The drawing under review shows one solid part. Ordinate dimensions are in mm from its lowest x, y, z. A direction names the side the tool comes from. Coordinates: 2 decimals unless noted, no trailing zeros. Loops run counter-clockwise (first coordinate to the right, second up) from the corner with the lowest first, then second, coordinate; pieces in that order, holes last. Notation, with made-up numbers: M -35.5,27 L -26.5,27 A23 ccw -26.5,61 Z; hole C 53.5,67 d5. An arc over 180 degrees is marked long. Answer as a JSON object with one key per item and string values. Group by question number.
1. Consider section A-A (z = 23). State the section outline as (x, y) points, then the cut area to 3 significant figures.
2. Insertion check: pin 1 (2 mm diameter, centred on x = 20, z = 36.5, fed in from +Y); pin 2 (0.9 mm diameter, centred on x = 35, y = 1, fed in from +Z); pin 3 (1.6 mm diameter, centred on y = 12, z = 30.5, fed in from -X). Each pin has a flat end and moves straight along its axis. Give the tip position at first contact, or say it passes through.
3. Machinability: for the marked faces 1 and 2, which of the approach directions +Z, -Z, +X, -X, +Y, -Y give a long, thin tool a straight path to every point of the face, cutting with its end or side? Answer none if there is none.
4. Draft analysis for pull direction Z (two halves, no side actions). For the marked faces 3, 4 and 5, state which applies: +Z half, -Z half, draft (parallel to the pull), parting line (faces both ways), or undercut.
5. To check wall thickness, follow probe 1 along Z at (x, y) = (14, 8.75); probe 2 along Z at (x, y) = (13.5, 11.5); probe 3 along X at (y, z) = (5, 30). State the ranges of each line that lie inside material, in increasing order.
6. Consider section B-B (x = 11). State the section outline as (y, z) points.
7. Consider section C-C (y = 1.25). State the section outline as (x, z) points, then the cut area to 3 significant figures.
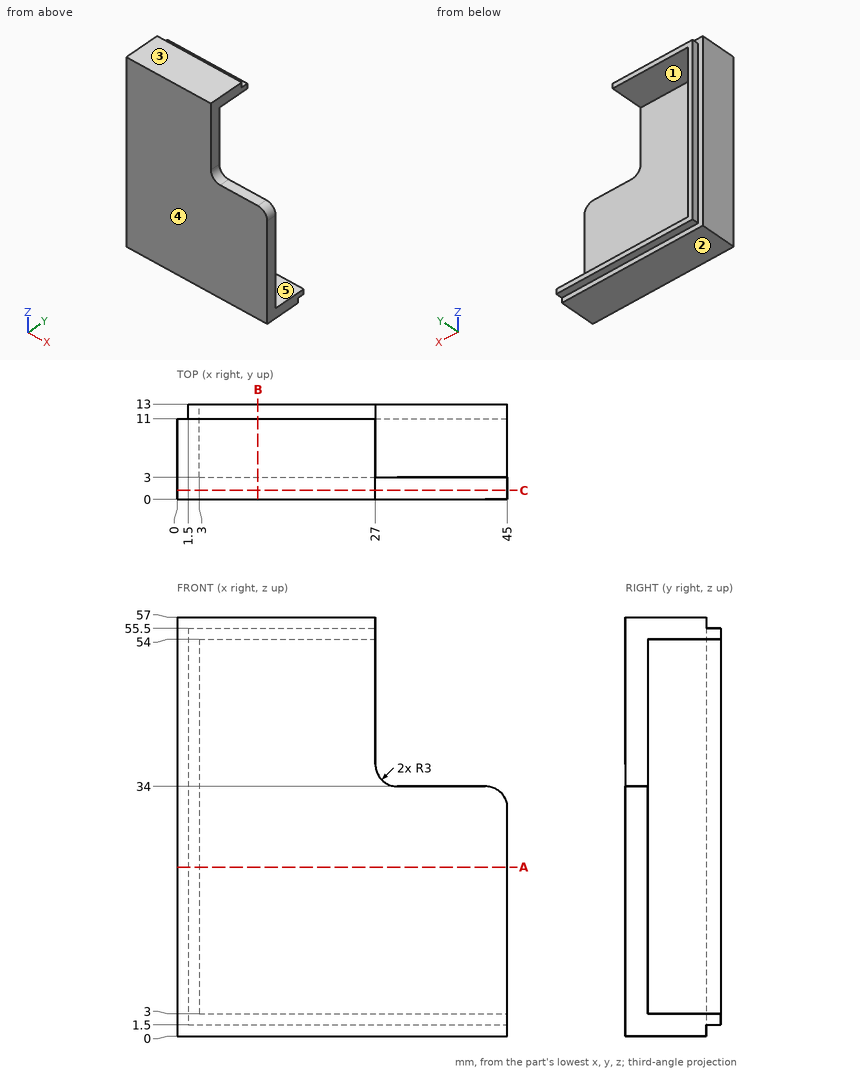
Findings below:
{
 "1": {"outline": "M 0,0 L 45,0 L 45,3 L 3,3 L 3,13 L 1.5,13 L 1.5,11 L 0,11 Z", "area": "162 mm^2"},
 "2": {"pin 1": "stops at y = 3", "pin 2": "stops at z = 34", "pin 3": "stops at x = 1.5"},
 "3": {"face 1": "+X, +Y", "face 2": "-Z, +X, -X, +Y, -Y"},
 "4": {"face 3": "+Z half", "face 4": "draft", "face 5": "undercut"},
 "5": {"probe 1": "z = 0 to 3, 54 to 57", "probe 2": "z = 1.5 to 3, 54 to 55.5", "probe 3": "x = 0 to 3"},
 "6": {"outline": "M 0,0 L 11,0 L 11,1.5 L 13,1.5 L 13,3 L 3,3 L 3,54 L 13,54 L 13,55.5 L 11,55.5 L 11,57 L 0,57 Z"},
 "7": {"outline": "M 0,0 L 45,0 L 45,31 A3 ccw 42,34 L 30,34 A3 cw 27,37 L 27,57 L 0,57 Z", "area": "2,150 mm^2"}
}
